Geometry check sheet. Reference: the model listing, model coordinates, mm. Give positions to 0.01 mm unless a question says otherwise; leave off trailing zeros. Write each loop counter-clockwise with the first axis right and the second up, starting at its lowest first coordinate (ties: lowest second). Pieces come first, ordered by that corner, then holes. Notation, with made-up numbers: (-40, 46.25) - (19, 46.25) arc R15 ccw to (19, 62.25) - close; hole circle Ø7 at (38.5, -23.5). An arc over 180 degrees is marked (long way). One line per question, with ' | ' between items. Start each with the question number.
Q1. Section check C-C on z = -25.4. Record the boundary of the cut face in (x, y), and give its area (3 significant figures).
Q2. Thickness scan on L1, parallel to Z at x = -15.6, y = 2.5; L2, parallel to X at y = 1.15, z = -25.4; L3, parallel to X at y = 3.5, z = -27. Record the ranges inside material, lowest first. Write a range as [from, to].
Q3. Section check B-B on y = 2.3. Record the boundary of the cut face in (x, z), and give its area (3 significant figures).
Q4. Section check A-A on x = 0. Record the boundary of the cut face in (y, z), and give its area (3 significant figures).
Q5. Section check D-D on x = 64.4. Record the boundary of the cut face in (y, z) (3 decimals), and give its area (4 significant figures).
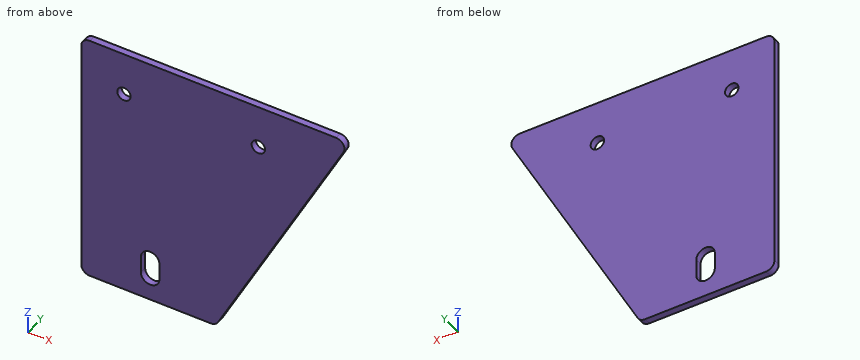
```python
from build123d import *

# Parameters (mm, degrees)
BOSS_EXTRUDE1_DEPTH = 4
SKETCH3_R           = 4
CUT_EXTRUDE1_DEPTH  = 5
FILLET1_R           = 5


with BuildPart() as part:
    # Sketch2 → Boss-Extrude1 (new body)
    with BuildSketch(Plane(origin=(0, 0, 0), x_dir=(1, 0, 0), z_dir=(0, 1, 0))):
        with BuildLine():
            Line((-41, 0), (110.666666667, 0))
            ThreePointArc((110.666666667, 0), (114.954131295, 2.427521223), (115.078431373, 7.352941176))
            Line((115.078431373, 7.352941176), (40.411764706, 147.352941176))
            ThreePointArc((40.411764706, 147.352941176), (38.572478777, 149.287464629), (36, 150))
            Line((36, 150), (-36, 150))
            ThreePointArc((-36, 150), (-39.535533906, 148.535533906), (-41, 145))
            Line((-41, 145), (-41, 0))
        make_face()
    extrude(amount=BOSS_EXTRUDE1_DEPTH)

    # Sketch3 → Cut-Extrude1 (cut, through all)
    with BuildSketch(Plane(origin=(0, 4, 0), x_dir=(1, 0, 0), z_dir=(0, 1, 0))):
        with Locations((-15.6, 25.4)):
            Circle(SKETCH3_R)
        with Locations((64.4, 25.4)):
            Circle(SKETCH3_R)
        with BuildLine():
            Line((5.5, 135), (5.5, 125))
            ThreePointArc((5.5, 125), (0, 119.5), (-5.5, 125))
            Line((-5.5, 125), (-5.5, 135))
            ThreePointArc((-5.5, 135), (0, 140.5), (5.5, 135))
        make_face()
    extrude(amount=-CUT_EXTRUDE1_DEPTH, mode=Mode.SUBTRACT)

    # Fillet1
    fillet1_edges = [part.edges().sort_by_distance(p)[0] for p in [
        (-41, 2, 0),
    ]]
    fillet(fillet1_edges, radius=FILLET1_R)


solid = part.part
```
Working result:
1) outline: (-41, 0) - (-19.6, 0) - (-19.6, 4) - (-41, 4) - close; (-11.6, 0) - (60.4, 0) - (60.4, 4) - (-11.6, 4) - close; (68.4, 0) - (105.45, 0) - (105.45, 4) - (68.4, 4) - close | area: 522 mm2
2) L1: z = [-150, -29.4], [-21.4, 0] | L2: x = [-41, -19.6], [-11.6, 60.4], [68.4, 105.45] | L3: x = [-41, -19.27], [-11.93, 60.73], [68.07, 104.6]
3) outline: (-41, -145) arc R5 ccw to (-36, -150) - (36, -150) arc R5 ccw to (40.41, -147.35) - (115.08, -7.35) arc R5 ccw to (110.67, 0) - (-36, 0) arc R5 ccw to (-41, -5) - close; hole circle Ø8 at (-15.6, -25.4); hole (-5.5, -135) arc R5.5 ccw to (5.5, -135) - (5.5, -125) arc R5.5 ccw to (-5.5, -125) - close; hole circle Ø8 at (64.4, -25.4) | area: 17,700 mm2
4) outline: (0, -150) - (4, -150) - (4, -140.5) - (0, -140.5) - close; (0, -119.5) - (4, -119.5) - (4, 0) - (0, 0) - close | area: 516 mm2
5) outline: (0, -102.375) - (4, -102.375) - (4, -29.4) - (0, -29.4) - close; (0, -21.4) - (4, -21.4) - (4, 0) - (0, 0) - close | area: 377.5 mm2
